from build123d import *

# Parameters (mm, degrees)
BOSS_EXTRUDE1_DEPTH  = 8
M2_CLEARANCE_HOLE2_D = 2.4
M2_CLEARANCE_HOLE1_D = 2.4


with BuildPart() as part:
    # Sketch1 → Boss-Extrude1 (new body)
    with BuildSketch(Plane.XY):
        with BuildLine():
            Line((0, 0), (8, 0))
            Line((8, 0), (8, 1))
            ThreePointArc((8, 1), (7.707106781, 1.707106781), (7, 2))
            Line((7, 2), (2, 2))
            Line((2, 2), (2, 6.6))
            ThreePointArc((2, 6.6), (1.707106781, 7.307106781), (1, 7.6))
            Line((1, 7.6), (-3, 7.6))
            ThreePointArc((-3, 7.6), (-3.707106781, 7.307106781), (-4, 6.6))
            Line((-4, 6.6), (-4, 5.6))
            Line((-4, 5.6), (0, 5.6))
            Line((0, 5.6), (0, 0))
        make_face()
    extrude(amount=BOSS_EXTRUDE1_DEPTH)

    # M2 Clearance Hole2 (through all)
    with Locations(Plane(origin=(0, 12, 0), x_dir=(1, 0, 0), z_dir=(0, 1, 0))):
        with Locations((5, -1.75)):
            Hole(M2_CLEARANCE_HOLE2_D / 2)

    # M2 Clearance Hole1 (through all)
    with Locations(Plane(origin=(0, 12, 0), x_dir=(1, 0, 0), z_dir=(0, 1, 0))):
        with Locations((5, -6.25)):
            Hole(M2_CLEARANCE_HOLE1_D / 2)


solid = part.part
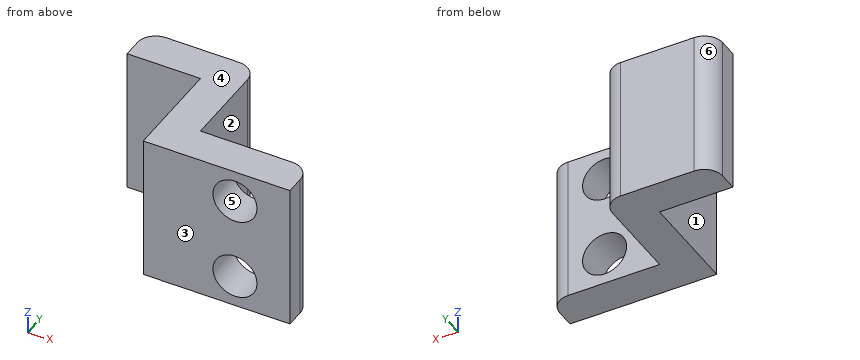
Input: part model. Units: mm. Frame: model coordinates. Face numbers are marked on the shaded views. A direction names the side the tool comes from. Coordinates: 2 decimals unless noted, no trailing zeros. Order: outer loops, then holes, each group sorted by start corner. A loop starts at its lowest first (then second) coordinate and runs counter-clockwise, first axis right, second up. Notation, with made-up numbers: M 35,87.5 L 74,87.5 A19 ccw 74,118.5 Z; hole C -3.5,-24 d10. An arc over 180 degrees is marked long. Write item = value, one per line. Start each with the question number.
(1) Line query: line 1 along Z through (x, y) = (5, 1.3); line 2 along Y through (x, z) = (-3, 1.25); line 3 along Y through (x, z) = (3, 3). Output: solid intervals per line, ascending. Write a range as [from, to].
(2) Section C-C on z = 3.25. Output: boundary loops of the cut face in (x, y), and give its area (3 significant figures).
(3) Pull-direction query (X, two-part tool) for the marked faces 4, 5 and 6; classes: released by +X, released by -X, zero draft, split by the parting line, or undercut.
(4) Reachability of the marked faces 1, 2 and 3 from +Z, -Z, +X, -X, +Y, -Y: full face, straight path, thin tool, end or side. Return the list, or none.
(5) Section D-D on y = 2.5. Output: boundary loops of the cut face in (x, z).
(6) First-contact query: P1, Ø3, axis at y = 2.5, z = 5.5, coming from the -X side; P2, Ø4.5, axis at x = -2.5, z = 5, coming from the -Y side; P3, Ø4, axis at x = 5, z = 1.75, coming from the +Y side. Flat tips, straight axial feed; report the tip coordinate or a pass-through.
(7) Section A-A on x = 5. Output: boundary loops of the cut face in (y, z).
(8) Section B-B on z = 5.5. Output: boundary loops of the cut face in (x, y), and give its area (3 significant figures).
Result set:
q1.line_1 = [0, 0.55], [2.95, 5.05], [7.45, 8]
q1.line_2 = [5.6, 7.6]
q1.line_3 = [0, 2]
q2.outline = M -4,5.6 L 0,5.6 L 0,0 L 8,0 L 8,1 A1 ccw 7,2 L 2,2 L 2,6.6 A1 ccw 1,7.6 L -3,7.6 A1 ccw -4,6.6 Z
q2.area = 34.6 mm²
q3.face_4 = zero draft
q3.face_5 = undercut
q3.face_6 = released by -X
q4.face_1 = +Z, -Z, -X, -Y
q4.face_2 = +Z, -Z, +X, +Y
q4.face_3 = +Z, -Z, +X, -X, -Y
q5.outline = M 0,0 L 2,0 L 2,8 L 0,8 Z
q6.P1 = 0
q6.P2 = 5.6
q6.P3 = 2
q7.outline = M 0,0 L 2,0 L 2,0.55 L 0,0.55 Z; M 0,2.95 L 2,2.95 L 2,5.05 L 0,5.05 Z; M 0,7.45 L 2,7.45 L 2,8 L 0,8 Z
q8.outline = M -4,5.6 L 0,5.6 L 0,0 L 4.06,0 L 4.06,2 L 2,2 L 2,6.6 A1 ccw 1,7.6 L -3,7.6 A1 ccw -4,6.6 Z; M 5.94,0 L 8,0 L 8,1 A1 ccw 7,2 L 5.94,2 Z
q8.area = 30.8 mm²
